```python
from build123d import *

# Parameters (mm, degrees)
F0_W     = 30
F0_H     = 20
F1_DEPTH = 2
F2_W     = 30
F2_H     = 20
F2_W_2   = 26
F2_H_2   = 16
F3_DEPTH = 30
F4_R     = 3.1
F5_DEPTH = 25
F6_W     = 50
F6_H     = 30
F6_W_2   = 26
F6_H_2   = 16
F7_DEPTH = 6
F9_DEPTH = 25


with BuildPart() as f1:
    # F0 (on Top) → F1 (new body)
    with BuildSketch(Plane.XY):
        with Locations((15, 10)):
            Rectangle(F0_W, F0_H)
    extrude(amount=F1_DEPTH)

    # F2 (on face) → F3 (join)
    with BuildSketch(Plane.XY.offset(2)):
        with Locations((15, 10)):
            Rectangle(F2_W, F2_H)
        with Locations((15, 10)):
            Rectangle(F2_W_2, F2_H_2, mode=Mode.SUBTRACT)
    extrude(amount=F3_DEPTH)

    # F4 (on face) → F5 (cut)
    with BuildSketch(Plane(origin=(0, 0, 0), x_dir=(1, 0, 0), z_dir=(0, 0, -1))):
        with Locations((8, -10)):
            Circle(F4_R)
        with Locations((22, -10)):
            Circle(F4_R)
    extrude(amount=-F5_DEPTH, mode=Mode.SUBTRACT)

    # F6 (on face) → F7 (join)
    with BuildSketch(Plane.XY.offset(32)):
        with Locations((15, 10)):
            Rectangle(F6_W, F6_H)
        with Locations((15, 10)):
            Rectangle(F6_W_2, F6_H_2, mode=Mode.SUBTRACT)
    extrude(amount=F7_DEPTH)

    # F8 (on face) → F9 (cut)
    with BuildSketch(Plane(origin=(0, 2, 0), x_dir=(-1, 0, 0), z_dir=(0, 1, 0))):
        with BuildLine():
            Line((-20, 38), (-20, 32))
            ThreePointArc((-20, 32), (-15, 27), (-10, 32))
            Line((-10, 32), (-10, 38))
            Line((-10, 38), (-20, 38))
        make_face()
    extrude(amount=-F9_DEPTH, mode=Mode.SUBTRACT)


solid = f1.part
```
Input: part model. Units: mm. Frame: model coordinates. A direction names the side the tool comes from. Round coordinates to 2 decimals unless told otherwise and drop trailing zeros. Loops run counter-clockwise (first coordinate to the right, second up) from the corner with the lowest first, then second, coordinate; pieces in that order, holes last. Notation, with made-up numbers: (36.5, 9.5) - (71.5, 9.5) arc R16 ccw to (71.5, 25.5) - close; hole circle Ø9 at (67, 50.5). An arc over 180 degrees is marked (long way). One line per item, written item: value. Start each with the question number.
(1) Section B-B, the plane z = 8.5. Return loops of the section in (x, y).
(2) Draft query along Y for faces 6 (the flat face through (15, 10, 2)), 7 (the flat face through (10, -1, 35)), 8 (the flat face through (15, 2, 20)), 9 (the flat face through (15, 20, 16)). Return one class per face: +Y half, -Y half, draft (parallel to the pull), parting line (faces both ways), or undercut.
(3) Ray query, line 1 (X direction, y = 10, z = 0.8); line 2 (X direction, y = 12.5, z = 24.5); line 3 (Y direction, x = 22, z = 1.05). Return the intervals inside material, ascending. Write a range as [from, to].
(4) Access query for faces 1 (the flat face through (2, 10, 20)), 2 (the flat face through (15, 0, 16)), 3 (the cylindrical face through (15, 1, 27)), 4 (the flat face through (30, 10, 16)), 5 (the flat face through (0, 10, 16)). Directions: +Z, -Z, +X, -X, +Y, -Y. A direction counts if a zero-diameter tool reaches every point of the face in a straight line with its end or side. Return the directions, or none.
(5) Section A-A, the plane x = 22. Return loops of the section in (y, z), plus the area to 3 significant figures.
(6) Section D-D, the plane x = 3.5. Return loops of the section in (y, z).
(7) Contact query for flat-ended pins moving along their axis: P1, Ø13, axis at y = 11, z = 13, coming from the +X side; P2, Ø5, axis at x = 9.5, y = 7, coming from the +Z side; P3, Ø8, axis at y = 11, z = 27.5, coming from the -X side; P4, Ø3.5, axis at x = 8, y = 10, coming from the -Z side. Output: stop coordinate, or through.
(8) Section C-C, the plane y = 10. Return loops of the section in (x, z), plus the area to 3 significant figures.
Results below:
1. outline: (0, 0) - (30, 0) - (30, 20) - (0, 20) - close; hole (2, 2) - (28, 2) - (28, 18) - (2, 18) - close
2. face 6: undercut
2. face 7: draft
2. face 8: undercut
2. face 9: +Y half
3. line 1: [0, 4.9], [11.1, 18.9], [25.1, 30]
3. line 2: [0, 2], [28, 30]
3. line 3: [0, 6.9], [13.1, 20]
4. face 1: +Z
4. face 2: -Z, +X, -X, -Y
4. face 3: +Z, -Y
4. face 4: -Z, +X, +Y, -Y
4. face 5: -Z, -X, +Y, -Y
5. outline: (-5, 32) - (0, 32) - (0, 0) - (6.9, 0) - (6.9, 2) - (2, 2) - (2, 38) - (-5, 38) - close; (13.1, 0) - (20, 0) - (20, 32) - (25, 32) - (25, 38) - (18, 38) - (18, 2) - (13.1, 2) - close
5. area: 232 mm^2
6. outline: (-5, 32) - (0, 32) - (0, 0) - (20, 0) - (20, 32) - (25, 32) - (25, 38) - (18, 38) - (18, 2) - (2, 2) - (2, 38) - (-5, 38) - close
7. P1: x = 30
7. P2: z = 2
7. P3: x = 0
7. P4: through
8. outline: (-10, 32) - (0, 32) - (0, 0) - (4.9, 0) - (4.9, 2) - (2, 2) - (2, 38) - (-10, 38) - close; (11.1, 0) - (18.9, 0) - (18.9, 2) - (11.1, 2) - close; (25.1, 0) - (30, 0) - (30, 32) - (40, 32) - (40, 38) - (28, 38) - (28, 2) - (25.1, 2) - close
8. area: 299 mm^2
